Autodesk Inventor part; units mm, degrees
ref_plane "Arbeitsebene1" through (12.5, 0, 0) normal (1, 0, 0) x (0, 1, 0)
ref_plane "XZ Plane" through (0, 0, 0) normal (0, 1, 0) x (-1, 0, 0)
ref_plane "XY Plane" through (0, 0, 0) normal (0, 0, 1) x (1, 0, 0)
sketch "Skizze1" plane through (0, 0, 0) normal (1, 0, 0) x (0, 1, 0)
  line L0 (0, 0) -> (13, 0) construction
  line L1 (0, 0) -> (13, 0) construction
  line L2 (2.5, 4) -> (0, 4)
  line L3 (0, 4) -> (0, -4)
  line L4 (0, -4) -> (2.5, -4)
  line L5 (2.5, -4) -> (2.5, 4)
  arc A0 (2.5, 4) -> (8.432, 3.6) centre (5.8166, 9) ccw
  arc A1 (8.432, -3.6) -> (2.5, -4) centre (5.8166, -9) ccw
  arc A2 (8.432, -3.6) -> (8.432, 3.6) centre (10.1755, 0) ccw
  circle A3 centre (10.1755, 0) radius 2
  dimension "d7" = 13
  dimension "d9" = 2.5
  dimension "d10" = 12
  dimension "d11" = 12
  dimension "d15" = 8
  dimension "d16" = 18
  dimension "d21" = 4
extrude "Extrusion1" add sketch "Skizze1" along normal blind 25 contours L5 L4 L3 L2
extrude "Extrusion2" add sketch "Skizze1" along normal blind 3 contours A0 A2 A1 L5
ref_plane "Arbeitsebene1" through (12.5, 0, 0) normal (1, 0, 0) x (0, 1, 0)
mirror "Spiegeln1" about plane through (12.5, 0, 0) normal (1, 0, 0) of "Extrusion2"
sketch "Skizze2" plane through (3, 2.5, 4) normal (0, 1, 0) x (1, 0, 0)
  line L0 (-3, 0) -> (-3, 8)
  line L1 (0, 0) -> (0, 8)
  point P0 (-3, 4)
  point P1 (4.5, 4)
  point P2 (14.5, 4)
  point P3 (-3, 4)
  point P4 (-3, 7.6)
  point P5 (-3, 0.4)
  point P6 (0, 7.6)
  point P7 (0, 0.4)
  dimension "d30" = 10
  dimension "d31" = 4.5
hole "Bohrung1" at (7.5, 2.5, 0) at (17.5, 2.5, 0) direction (0, -1, 0) diameter 3.5 depth 2.5
properties part number "kipphebellagerbock"
The model under review builds one solid part; all positions refer to its coordinate system, in mm. A direction names the side the tool comes from. Round coordinates to 2 decimals unless told otherwise and drop trailing zeros. Loops run counter-clockwise (first coordinate to the right, second up) from the corner with the lowest first, then second, coordinate; pieces in that order, holes last. Notation, with made-up numbers: (47.25, 13.25) - (57.25, 13.25) arc R17 cw to (57.25, 43.25) - close; hole circle Ø1 at (-3.5, 26). An arc over 180 degrees is marked (long way). Use a Markdown table: item, result. Add a question column.
Q1. Add section B-B (y = 1.25). State the section outline as (x, z) points, plus the area to 3 significant figures.
Q2. Machinability: for faces 5 (the face through (1.479, 12.083, -0.601)), 6 (the face through (3, 7, 0)), which of the approach directions +Z, -Z, +X, -X, +Y, -Y give a long, thin tool a straight path to every point of the face, cutting with its end or side? Answer none if there is none.
Q3. Insertion check: pin 1 Ø4 at (x, z) = (12, 0.5) entering from +Y. The pin has a flat end and moves straight along its axis. Give the tip position at first contact, or say it passes through.
Q4. For probe 1 along X at (y, z) = (0.7, 0); probe 2 along X at (y, z) = (11.25, -3.5); probe 3 along Z at (x, y) = (7.5, 0.8), list the stretches that pass through material, from the lowest coordinate up.
Q5. The part is to be moulded in two halves that separate along X. For faces 1 (the face through (0, 5, 0)), 2 (the face through (12, 1, 4)), 3 (the face through (25, 6, 0)), 4 (the face through (15.765, 1.232, -0.228)), say which applies: pulls with the +X half, pulls with the -X half, needs draft (parallel to the pull), parting line crosses it, or undercut.
Q6. Add section D-D (y = 5). State the section outline as (x, z) points.
Q7. Add section A-A (x = 7.5). State the section outline as (y, z) points.
Q8. Add section C-C (z = 0). State the section outline as (x, y) points.
Worked answers:
| question | item | result |
|---|---|---|
| 1 | outline | (0, -4) - (25, -4) - (25, 4) - (0, 4) - close; hole circle Ø3.5 at (7.5, 0); hole circle Ø3.5 at (17.5, 0) |
| 1 | area | 181 mm² |
| 2 | face 5 | +X, -X |
| 2 | face 6 | +Z, -Z, +Y |
| 3 | pin 1 | y = 2.5 |
| 4 | probe 1 | 0 to 5.75, 9.25 to 15.75, 19.25 to 25 |
| 4 | probe 2 | 0 to 3, 22 to 25 |
| 4 | probe 3 | -4 to -1.75, 1.75 to 4 |
| 5 | face 1 | pulls with the -X half |
| 5 | face 2 | needs draft |
| 5 | face 3 | pulls with the +X half |
| 5 | face 4 | undercut |
| 6 | outline | (0, -3.06) - (3, -3.06) - (3, 3.06) - (0, 3.06) - close; (22, -3.06) - (25, -3.06) - (25, 3.06) - (22, 3.06) - close |
| 7 | outline | (0, -4) - (2.5, -4) - (2.5, -1.75) - (0, -1.75) - close; (0, 1.75) - (2.5, 1.75) - (2.5, 4) - (0, 4) - close |
| 8 | outline | (0, 0) - (5.75, 0) - (5.75, 2.5) - (3, 2.5) - (3, 8.18) - (0, 8.18) - close; (0, 12.18) - (3, 12.18) - (3, 14.18) - (0, 14.18) - close; (9.25, 0) - (15.75, 0) - (15.75, 2.5) - (9.25, 2.5) - close; (19.25, 0) - (25, 0) - (25, 8.18) - (22, 8.18) - (22, 2.5) - (19.25, 2.5) - close; (22, 12.18) - (25, 12.18) - (25, 14.18) - (22, 14.18) - close |
